Read the model definition and answer for the solid it produces. Units are mm, in the model's axes. A direction names the side the tool comes from. Coordinates: 2 decimals unless noted, no trailing zeros. Order: outer loops, then holes, each group sorted by start corner. A loop starts at its lowest first (then second) coordinate and runs counter-clockwise, first axis right, second up. Notation, with made-up numbers: (-12, -4) - (-8, -4) arc R10 cw to (-8, 5) - close; hole circle Ø6 at (11, -28.5). An arc over 180 degrees is marked (long way). Use one line per item in the form item = value.
```python
from build123d import *

# Parameters (mm, degrees)
F0_W     = 8
F0_H     = 16
F0_W_2   = 4.4
F0_H_2   = 12.4
F1_DEPTH = 2
F2_W     = 8
F2_H     = 16
F3_DEPTH = 1.2
F4_R     = 2.5
F5_DEPTH = 1.8
F7_DEPTH = 2
F8_R     = 1.25
F9_DEPTH = 1.5


with BuildPart() as f1:
    # F0 (on Top) → F1 (new body)
    with BuildSketch(Plane.XY):
        with Locations((1.777131, -13.520962)):
            Rectangle(F0_W, F0_H)
        with Locations((1.777131, -13.520962)):
            Rectangle(F0_W_2, F0_H_2, mode=Mode.SUBTRACT)
    extrude(amount=F1_DEPTH)

    # F2 (on face) → F3 (join)
    with BuildSketch(Plane.XY.offset(2)):
        with Locations((1.777131, -13.520962)):
            Rectangle(F2_W, F2_H)
    extrude(amount=F3_DEPTH)

    # F4 (on face) → F5 (join)
    with BuildSketch(Plane.XY.offset(3.2)):
        with Locations((1.777131, -9.520962)):
            Circle(F4_R)
        with Locations((1.777131, -17.520962)):
            Circle(F4_R)
    extrude(amount=F5_DEPTH)

    # F6 (on face) → F7 (join)
    with BuildSketch(Plane(origin=(0, 0, 2), x_dir=(1, 0, 0), z_dir=(0, 0, -1))):
        with BuildLine():
            ThreePointArc((1.027131, 13.520962), (1.777131, 14.270962), (2.527131, 13.520962))
            Line((2.527131, 13.520962), (3.277131, 13.520962))
            ThreePointArc((3.277131, 13.520962), (1.777131, 15.020962), (0.277131, 13.520962))
            Line((0.277131, 13.520962), (1.027131, 13.520962))
        make_face()
        with BuildLine():
            Line((3.277131, 13.520962), (2.527131, 13.520962))
            ThreePointArc((2.527131, 13.520962), (1.777131, 12.770962), (1.027131, 13.520962))
            Line((1.027131, 13.520962), (0.277131, 13.520962))
            ThreePointArc((0.277131, 13.520962), (1.777131, 12.020962), (3.277131, 13.520962))
        make_face()
    extrude(amount=F7_DEPTH)

    # F8 (on face) → F9 (cut)
    with BuildSketch(Plane(origin=(0, 0, 2), x_dir=(1, 0, 0), z_dir=(0, 0, -1))):
        with Locations((1.777131, 17.370962)):
            Circle(F8_R)
        with Locations((1.777131, 9.670962)):
            Circle(F8_R)
    extrude(amount=-F9_DEPTH, mode=Mode.SUBTRACT)


solid = f1.part
```
(1) Section C-C, the plane y = -15.5 is taken. Write down the section's boundary in (x, z).
Answer list:
outline = (-2.22, 0) - (-0.42, 0) - (-0.42, 2) - (3.98, 2) - (3.98, 0) - (5.78, 0) - (5.78, 3.2) - (3.25, 3.2) - (3.25, 5) - (0.31, 5) - (0.31, 3.2) - (-2.22, 3.2) - close
(2) The mould has two halves that part along X. Classify faces 4 (the flat face through (5.777, -14, 2)), 5 (the flat face through (2, -17, 5)), 6 (the flat face through (-2.223, -14, 2)), 7 (the flat face through (2, -19.721, 1)): +X half, -X half, draft (parallel to the pull), parting line (faces both ways), or undercut.
Answer list:
face_4 = +X half
face_5 = draft
face_6 = -X half
face_7 = undercut
(3) Section B-B, the plane x = 2.75 is taken. Write down the section's boundary in (y, z), then the cut area to 3 significant figures.
Answer list:
outline = (-21.52, 0) - (-19.72, 0) - (-19.72, 2) - (-18.16, 2) - (-18.16, 3.5) - (-16.59, 3.5) - (-16.59, 2) - (-14.66, 2) - (-14.66, 0) - (-12.38, 0) - (-12.38, 2) - (-10.46, 2) - (-10.46, 3.5) - (-8.89, 3.5) - (-8.89, 2) - (-7.32, 2) - (-7.32, 0) - (-5.52, 0) - (-5.52, 3.2) - (-7.22, 3.2) - (-7.22, 5) - (-11.82, 5) - (-11.82, 3.2) - (-15.22, 3.2) - (-15.22, 5) - (-19.82, 5) - (-19.82, 3.2) - (-21.52, 3.2) - close
area = 42.8 mm2
(4) Straight lines are drawn through the part: L1, parallel to X at y = -18, z = 1; L2, parallel to Y at x = 1.5, z = 2.25; L3, parallel to Z at x = 3.75, y = -10.25. For each, find the intervals that lie inside material, in ascending order.
Answer list:
L1 = -2.22 to -0.42, 3.98 to 5.78
L2 = -21.52 to -18.59, -16.15 to -10.89, -8.45 to -5.52
L3 = 2 to 5
(5) Which of the six approach directions +Z, -Z, +X, -X, +Y, -Y give full straight-line access (tool end or side, diameter ignored) to faces 1 (the flat face through (-1, -13, 0)), 2 (the flat face through (1, -12, 2)), 3 (the cylindrical face through (1.452, -7.042, 4.087))?
Answer list:
face_1 = -Z, +X, -X, +Y, -Y
face_2 = -Z
face_3 = +Z
(6) Section D-D, the plane z = 2.7 is taken. Write down the section's boundary in (x, y).
Answer list:
outline = (-2.22, -21.52) - (5.78, -21.52) - (5.78, -5.52) - (-2.22, -5.52) - close; hole circle Ø2.5 at (1.78, -17.37); hole circle Ø2.5 at (1.78, -9.67)
(7) Given pin 1 Ø1.2 at (x, y) = (2, -17.5) entering from -Z; pin 2 Ø1.4 at (x, y) = (1.78, -13.52) entering from +Z, each flat-ended and moving along its own axis, determine where each tip first touches the part or whether it passes through.
Answer list:
pin_1 = 3.5
pin_2 = 3.2
(8) Section A-A, the plane z = 0.5 is taken. Write down the section's boundary in (x, y).
Answer list:
outline = (-2.22, -21.52) - (5.78, -21.52) - (5.78, -5.52) - (-2.22, -5.52) - close; circle Ø3 at (1.78, -13.52); hole (-0.42, -19.72) - (3.98, -19.72) - (3.98, -7.32) - (-0.42, -7.32) - close; hole circle Ø1.5 at (1.78, -13.52)
